CAD build for the part. Positions are in the model's coordinates, mm. Face numbers are marked on the shaded views. A direction names the side the tool comes from. Coordinates: 2 decimals unless noted, no trailing zeros. Loops run counter-clockwise (first coordinate to the right, second up) from the corner with the lowest first, then second, coordinate; pieces in that order, holes last. Notation, with made-up numbers: (-31, -13) -> (-19, -13) arc R9 ccw to (-19, -3) -> close; hole circle Ø10 at (88, -33). An arc over 180 degrees is marked (long way). Write each question's results on one line, items separated by ' | '.
from build123d import *

# Parameters (mm, degrees)
SKETCH1_R           = 17.5
BOSS_EXTRUDE1_DEPTH = 30
SKETCH2_W           = 22.36
SKETCH2_H           = 22
CUT_EXTRUDE1_DEPTH  = 30
BOSS_EXTRUDE2_DEPTH = 20


with BuildPart() as part:
    # Sketch1 → Boss-Extrude1 (new body)
    with BuildSketch(Plane(origin=(0, 0, 0), x_dir=(1, 0, 0), z_dir=(0, 1, 0))):
        with Locations(Location((0, 0, 0), (0, 0, 270))):
            Circle(SKETCH1_R)
    extrude(amount=BOSS_EXTRUDE1_DEPTH)

    # Sketch2 → Cut-Extrude1 (cut)
    with BuildSketch(Plane(origin=(0, 0, 0), x_dir=(0, 0, -1), z_dir=(1, 0, 0))):
        with Locations((0, 15)):
            Rectangle(SKETCH2_W, SKETCH2_H)
    extrude(amount=-CUT_EXTRUDE1_DEPTH, mode=Mode.SUBTRACT)

    # Sketch3 → Boss-Extrude2 (add)
    with BuildSketch(Plane.XZ):
        with BuildLine():
            Line((-0.5, -1.414213562), (-0.5, -0.4))
            Line((-0.5, -0.4), (0.5, -0.4))
            Line((0.5, -0.4), (0.5, -1.414213562))
            ThreePointArc((0.5, -1.414213562), (1.224744871, -0.866025404), (1.5, 0))
            ThreePointArc((1.5, 0), (-0.866025404, 1.224744871), (-0.5, -1.414213562))
        make_face()
        with BuildLine():
            Line((0.5, -0.4), (-0.5, -0.4))
            Line((-0.5, -0.4), (-0.5, -1.414213562))
            ThreePointArc((-0.5, -1.414213562), (0, -1.5), (0.5, -1.414213562))
            Line((0.5, -1.414213562), (0.5, -0.4))
        make_face()
        with BuildLine():
            ThreePointArc((0.5, -1.414213562), (0, -1.5), (-0.5, -1.414213562))
            Line((-0.5, -1.414213562), (-0.5, -2.6))
            Line((-0.5, -2.6), (0.5, -2.6))
            Line((0.5, -2.6), (0.5, -1.414213562))
        make_face()
    extrude(amount=BOSS_EXTRUDE2_DEPTH)


solid = part.part
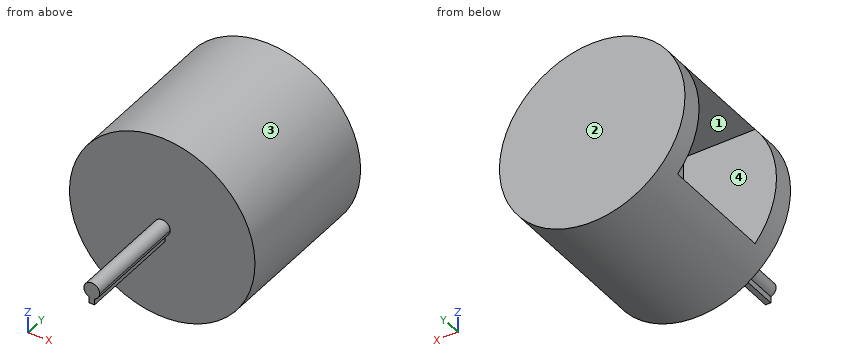
1) Slice it at C-C (x = 13.5). Write the cut outline in (y, z).
Outcome:
outline: (0, -11.14) -> (30, -11.14) -> (30, 11.14) -> (0, 11.14) -> close
2) Which spindle directions (+Z, -Z, +X, -X, +Y, -Y) get a long thin tool onto all of the face, cutting with end or side? Do the marked faces 3 and 4. Say none if no direction does.
Outcome:
face 3: +Y, -Y | face 4: -X
3) Two-plate mould, pull along Y, no slides. Class the marked faces 1 and 2: pulls with the +Y half, pulls with the -Y half, needs draft (parallel to the pull), parting line crosses it, or undercut.
Outcome:
face 1: undercut | face 2: pulls with the +Y half
4) Pin check, flat tips, straight feed: pin 1 (15 mm diameter, centred on x = -9, y = 13, fed in from +Z); pin 2 (1.5 mm diameter, centred on y = 12.5, z = -1.5, fed in from -X); pin 3 (12 mm diameter, centred on y = 13.5, z = 11.5, fed in from -X). Stop position of each tip, or through.
Outcome:
pin 1: stops at z = 17.44 | pin 2: stops at x = 0 | pin 3: stops at x = -13.46
5) Drill centre lines: L1, parallel to Y at x = -2, z = 3; L2, parallel to Z at x = -5, y = 22; L3, parallel to Y at x = 3.5, z = 2.5. Where is each one in solid material? Low to high. Write a range as from..to.
Outcome:
L1: y = 0..4, 26..30 | L2: z = -16.77..-11.18, 11.18..16.77 | L3: y = 0..30
6) Slice it at B-B (y = 22.5). Write the cut outline in (x, z).
Outcome:
outline: (-13.46, -11.18) arc R17.5 ccw (long way) to (-13.46, 11.18) -> (0, 11.18) -> (0, -11.18) -> close
7) Slice it at A-A (z = 10.5). Write the cut outline in (x, y).
Outcome:
outline: (-14, 0) -> (14, 0) -> (14, 30) -> (-14, 30) -> (-14, 26) -> (0, 26) -> (0, 4) -> (-14, 4) -> close
